Autodesk Inventor part; units mm, degrees
ref_plane "YZ Plane" through (0, 0, 0) normal (1, 0, 0) x (0, 1, 0)
ref_plane "XZ Plane" through (0, 0, 0) normal (0, 1, 0) x (-1, 0, 0)
ref_plane "XY Plane" through (0, 0, 0) normal (0, 0, 1) x (1, 0, 0)
sketch "Sketch1" plane through (0, 0, 0) normal (0, 1, 0) x (-1, 0, 0)
  line L0 (0, 0) -> (-37, 0)
  line L1 (-37, 0) -> (-37, 37)
  line L2 (-37, 37) -> (0, 37)
  line L3 (0, 37) -> (0, 0)
  circle A0 centre (-18.5, 18.5) radius 15.5
  point P0 (-18.5, 0)
  dimension "d0" = 37
  dimension "d1" = 37
  dimension "d2" = 18.5
  dimension "d3" = 18.5
  dimension "d4" = 31
extrude "Extrusion1" add sketch "Sketch1" against normal blind 20
sketch "Sketch3" plane through (0, 0, 37) normal (0, 0, 1) x (1, 0, 0)
  circle A0 centre (20.5, -10) radius 4.5
  point P0 (0, 0)
  dimension "d8" = 9
extrude "Extrusion2" cut sketch "Sketch3" against normal blind 5
sketch "Sketch4" plane through (37, 0, 0) normal (0, 0, -1) x (-1, 0, 0)
  circle A0 centre (16.5, -10) radius 4.5
  circle A1 centre (16.5, -10) radius 2.5
  point P0 (37, 0)
  dimension "d11" = 5
extrude "Extrusion3" cut sketch "Sketch4" against normal blind 5 contours A1
sketch "Sketch5" plane through (0, 0, 37) normal (0, 0, 1) x (1, 0, 0)
  line L0 (37, 0) -> (0, 0)
  line L1 (0, -20) -> (37, -20)
  line L2 (0, 0) -> (37, 0)
  line L3 (37, 0) -> (37, -20)
  line L4 (37, -20) -> (0, -20)
  line L5 (0, -20) -> (0, 0)
  line L6 (0, 0) -> (0, -20)
  line L7 (0, 0) -> (37, 0)
  line L8 (37, 0) -> (37, -20)
  line L9 (37, -20) -> (0, -20)
  line L10 (0, -20) -> (0, 0)
  circle A0 centre (20.5, -10) radius 4.5
extrude "Extrusion4" add sketch "Sketch5" along normal blind 2
sketch "Sketch6" plane through (0, 0, 39) normal (0, 0, 1) x (1, 0, 0)
  line L0 (0, 0) -> (0, -20)
  line L1 (0, -20) -> (37, -20)
  line L2 (0, 0) -> (37, 0)
  line L3 (37, 0) -> (37, -20)
  line L4 (37, -20) -> (0, -20)
  line L5 (0, -20) -> (0, 0)
  circle A0 centre (20.5, -10) radius 2.5
extrude "Extrusion5" add sketch "Sketch6" along normal blind 5
equation "\"d0\" = d1"
properties part number "welco mount v02"
Model file for the job. Use its own axes, mm. A direction names the side the tool comes from. Give positions to 0.01 mm unless a question says otherwise; leave off trailing zeros. Loops run counter-clockwise (first coordinate to the right, second up) from the corner with the lowest first, then second, coordinate; pieces in that order, holes last. Notation, with made-up numbers: (27.25, 74.25) -> (76.25, 74.25) arc R24 cw to (76.25, 84.25) -> close; hole circle Ø6 at (-18, 49.5). An arc over 180 degrees is marked (long way). Use CSV: the item, a comma, the result in double quotes. Start each with the question number.
1) Mould opens along X. For faces 3 (the flat face through (37, -10, 22)), 4 (the flat face through (18, -20, 36)), 5 (the cylindrical face through (19, -8, 41)) say: released by +X, released by -X, zero draft, split by the parting line, or undercut.
2) Slice it at D-D on y = -12. Give the cut face in (x, z).
3) Slice it at B-B on y = -4.25. Give the cut face in (x, z).
4) Slice it at C-C on x = 18.5. Give the cut face in (y, z), plus the area to 3 significant figures.
5) Slice it at A-A on z = 18.5. Give the cut face in (x, y), plus the area to 3 significant figures.
6) Wall check: line 1 (X direction, y = -10, z = 2.95); line 2 (Z direction, x = 18.5, y = -13); line 3 (Y direction, x = 20.5, z = 37). Give the ranges that are in metal, low to high.
7) Tool access for faces 1 (the cylindrical face through (24.792, -11.352, 36.455)), 2 (the flat face through (18, -12, 0)): list every direction of +Z, -Z, +X, -X, +Y, -Y with a clear straight run to the whole face (end or side of a thin tool).
Computed values:
1,face 3,"released by +X"
1,face 4,"zero draft"
1,face 5,"undercut"
2,outline,"(0, 0) -> (19, 0) -> (19, 3.01) arc R15.5 cw to (16.47, 33.87) -> (16.47, 39) -> (19, 39) -> (19, 44) -> (0, 44) -> close; (22, 0) -> (37, 0) -> (37, 44) -> (22, 44) -> (22, 39) -> (24.53, 39) -> (24.53, 32.78) arc R15.5 cw to (22, 3.4) -> close"
3,outline,"(0, 0) -> (37, 0) -> (37, 44) -> (0, 44) -> close; hole circle Ø31 at (18.5, 18.5)"
4,outline,"(-20, 0) -> (-11.5, 0) -> (-11.5, 3) -> (-20, 3) -> close; (-20, 34) -> (-14.03, 34) -> (-14.03, 39) -> (-11.5, 39) -> (-11.5, 44) -> (-20, 44) -> close; (-8.5, 0) -> (0, 0) -> (0, 3) -> (-8.5, 3) -> close; (-8.5, 39) -> (-5.97, 39) -> (-5.97, 34) -> (0, 34) -> (0, 44) -> (-8.5, 44) -> close"
4,area,"196 mm^2"
5,outline,"(0, -20) -> (3, -20) -> (3, 0) -> (0, 0) -> close; (34, -20) -> (37, -20) -> (37, 0) -> (34, 0) -> close"
5,area,"120 mm^2"
6,line 1,"x = 0 to 18, 23 to 37"
6,line 2,"z = 0 to 3, 39 to 44"
6,line 3,"y = -20 to -14.5, -5.5 to 0"
7,face 1,"none"
7,face 2,"-Z, +X, -X, +Y, -Y"
